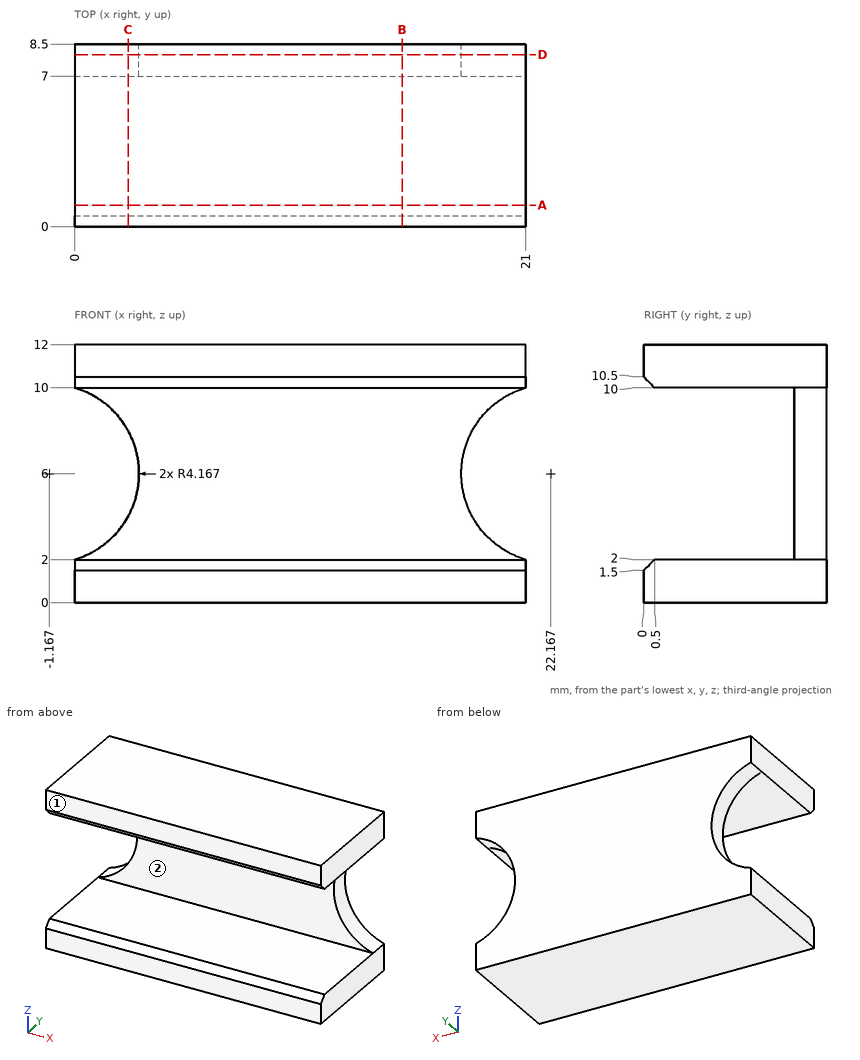
Verification items for this drawing (mm, ordinates from the low corner). A direction names the side the tool comes from. Coordinates: 2 decimals unless noted, no trailing zeros. Loops run counter-clockwise (first coordinate to the right, second up) from the corner with the lowest first, then second, coordinate; pieces in that order, holes last.
Item 1: Access from +Z, -Z, +X, -X, +Y, -Y to the whole of each face (thin tool, end or side, straight path). Record for the marked faces 1 and 2.
Item 2: Sectioned sample at B-B, the plane x = 15.25. Record the boundary of the cut face in (y, z).
Item 3: Sectioned sample at C-C, the plane x = 2.5. Record the boundary of the cut face in (y, z).
Item 4: Sectioned sample at A-A, the plane y = 1. Record the boundary of the cut face in (x, z).
Item 5: Go/stop test with flat-tipped pins: pin 1 Ø4 at (x, z) = (15.5, 7) entering from -Y; pin 2 Ø1 at (y, z) = (5, 3.5) entering from -X. Record where each tip stops, or that it passes through.
Item 6: Thickness scan on line 1 (Z direction, x = 3.75, y = 0.75); line 2 (Y direction, x = 8.75, z = 4.75); line 3 (X direction, y = 8, z = 2.75). Record the ranges inside material, lowest first.
Item 7: Sectioned sample at D-D, the plane y = 8. Record the boundary of the cut face in (x, z).
Check result:
1. face 1: +Z, -Z, +X, -X, -Y
1. face 2: +X, -X, -Y
2. outline: (0, 0) - (8.5, 0) - (8.5, 12) - (0, 12) - (0, 10.5) - (0.5, 10) - (7, 10) - (7, 2) - (0.5, 2) - (0, 1.5) - close
3. outline: (0, 0) - (8.5, 0) - (8.5, 4.02) - (7, 4.02) - (7, 2) - (0.5, 2) - (0, 1.5) - close; (0, 10.5) - (0.5, 10) - (7, 10) - (7, 7.98) - (8.5, 7.98) - (8.5, 12) - (0, 12) - close
4. outline: (0, 0) - (21, 0) - (21, 2) - (0, 2) - close; (0, 10) - (21, 10) - (21, 12) - (0, 12) - close
5. pin 1: stops at y = 7
5. pin 2: passes through
6. line 1: z = 0 to 2, 10 to 12
6. line 2: y = 7 to 8.5
6. line 3: x = 1.44 to 19.56
7. outline: (0, 0) - (21, 0) - (21, 2) arc R4.17 cw to (21, 10) - (21, 12) - (0, 12) - (0, 10) arc R4.17 cw to (0, 2) - close
